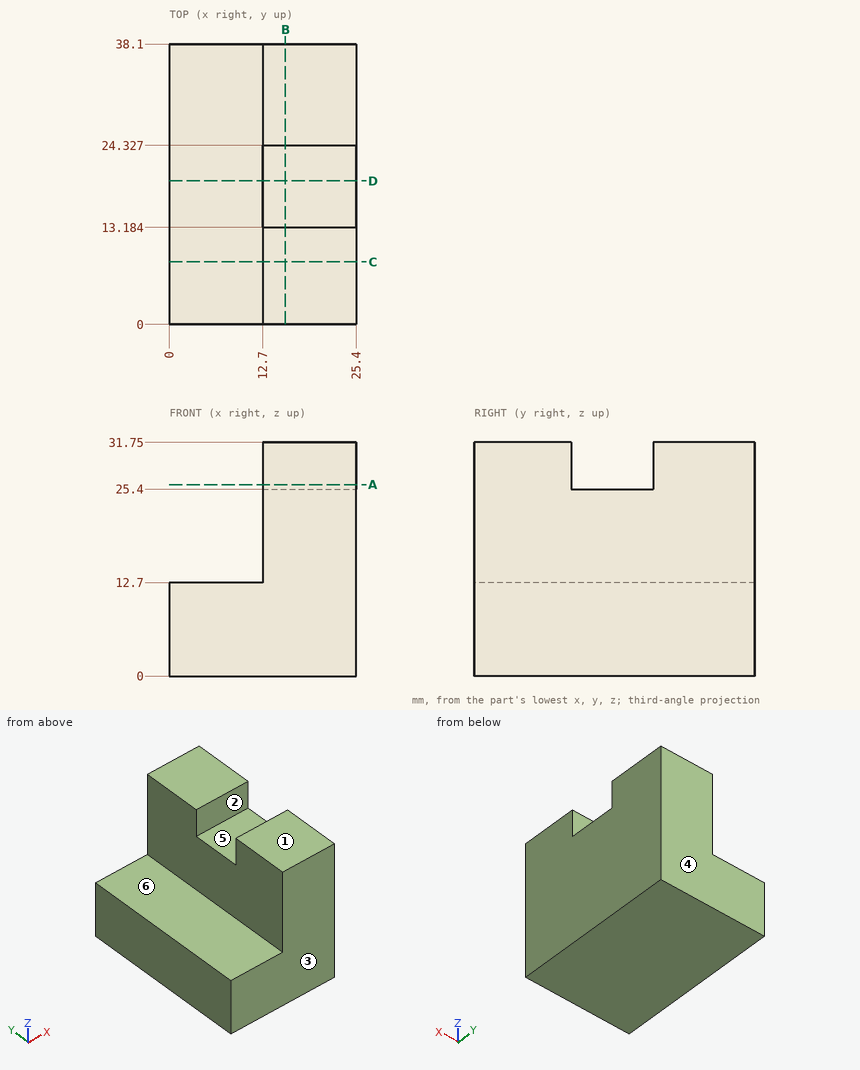
Study the drawing (mm; zero at the part's minimum x, y, z) and answer. A direction names the side the tool comes from. Round coordinates to 2 decimals unless told otherwise and drop trailing zeros. Write each loop counter-clockwise with the first axis right and the second up, starting at its lowest first coordinate (ties: lowest second). Pieces come first, ordered by that corner, then holes. Notation, with made-up numbers: (9.5, 13) -> (53.5, 13) arc R32 ccw to (53.5, 40) -> close; hole circle Ø1 at (-25, -14). An arc over 180 degrees is marked (long way). Use CSV: the item, a comma, the result in double quotes. Start each with the question number.
(1) Consider L1, parallel to Y at x = 22.25, z = 26; L2, parallel to X at y = 23, z = 25; L3, parallel to Z at x = 2.25, y = 14. Determine where each line is inside the solid, lowest interval first. Write a range as from..to.
(2) The mould has two halves that part along Y. Classify the marked faces 1, 2 and 3: released by +Y, released by -Y, zero draft, split by the parting line, or undercut.
(3) Section C-C on y = 8.5 is taken. Give the vertices of the cut face in (x, z).
(4) Section B-B on x = 15.75 is taken. Give the vertices of the cut face in (y, z), then the cut area to 3 significant figures.
(5) Which of the six approach directions +Z, -Z, +X, -X, +Y, -Y give full straight-line access (tool end or side, diameter ignored) to the marked faces 4, 5 and 6?
(6) Section D-D on y = 19.5 is taken. Give the vertices of the cut face in (x, z), then the cut area to 3 significant figures.
(7) Each of these flat-tipped pins is pushed along its axis until it touches: pin 1 (10 mm diameter, centred on x = 6, y = 16, fed in from +Z); pin 2 (5.5 mm diameter, centred on y = 11.5, z = 18, fed in from -X). Where does it stop, or does it pass through?
(8) Section A-A on z = 26 is taken. Give the vertices of the cut face in (x, y), then the cut area to 3 significant figures.
A:
1,L1,"y = 0..13.18, 24.33..38.1"
1,L2,"x = 12.7..25.4"
1,L3,"z = 0..12.7"
2,face 1,"zero draft"
2,face 2,"undercut"
2,face 3,"released by -Y"
3,outline,"(0, 0) -> (25.4, 0) -> (25.4, 31.75) -> (12.7, 31.75) -> (12.7, 12.7) -> (0, 12.7) -> close"
4,outline,"(0, 0) -> (38.1, 0) -> (38.1, 31.75) -> (24.33, 31.75) -> (24.33, 25.4) -> (13.18, 25.4) -> (13.18, 31.75) -> (0, 31.75) -> close"
4,area,"1,140 mm²"
5,face 4,"+Z, -Z, +X, -X, +Y"
5,face 5,"+Z, +X, -X"
5,face 6,"+Z, -X, +Y, -Y"
6,outline,"(0, 0) -> (25.4, 0) -> (25.4, 25.4) -> (12.7, 25.4) -> (12.7, 12.7) -> (0, 12.7) -> close"
6,area,"484 mm²"
7,pin 1,"stops at z = 12.7"
7,pin 2,"stops at x = 12.7"
8,outline,"(12.7, 0) -> (25.4, 0) -> (25.4, 13.18) -> (12.7, 13.18) -> close; (12.7, 24.33) -> (25.4, 24.33) -> (25.4, 38.1) -> (12.7, 38.1) -> close"
8,area,"342 mm²"
